The model under review builds one solid part; all positions refer to its coordinate system, in mm. A direction names the side the tool comes from. Coordinates: 2 decimals unless noted, no trailing zeros. Order: outer loops, then holes, each group sorted by start corner. A loop starts at its lowest first (then second) coordinate and runs counter-clockwise, first axis right, second up. Notation, with made-up numbers: (25.5, 27.5) -> (36.5, 27.5) arc R33 ccw to (36.5, 58.5) -> close; hole circle Ø1 at (24.5, 5.5). An arc over 180 degrees is marked (long way). Put each result on its own line as item: value.
from build123d import *

# Parameters (mm, degrees)
SKETCH1_R           = 1.905
BOSS_EXTRUDE1_DEPTH = 0.8001
CIRPATTERN1_COUNT   = 3
SKETCH2_R           = 2.54
CUT_EXTRUDE1_DEPTH  = 2.6002
FILLET1_R           = 6.35


with BuildPart() as part:
    # Sketch1 → Boss-Extrude1 (new body, symmetric)
    with BuildSketch(Plane(origin=(0, 0, 0), x_dir=(1, 0, 0), z_dir=(0, 1, 0))):
        with BuildLine():
            Line((-5.08, 17.78), (-5.08, 0))
            Line((-5.08, 0), (5.08, 0))
            Line((5.08, 0), (5.08, 17.78))
            ThreePointArc((5.08, 17.78), (0, 22.86), (-5.08, 17.78))
        make_face()
        with Locations((0, 17.78)):
            Circle(SKETCH1_R, mode=Mode.SUBTRACT)
    boss_extrude1 = extrude(amount=BOSS_EXTRUDE1_DEPTH, both=True)

    # CirPattern1: Boss-Extrude1 ×3 about axis
    cirpattern1_axis = Axis((0, 0, 0), (0, 1, 0))
    for i in range(1, CIRPATTERN1_COUNT):
        add(boss_extrude1.rotate(cirpattern1_axis, i * 360 / CIRPATTERN1_COUNT))

    # Sketch2 → Cut-Extrude1 (cut, through all)
    with BuildSketch(Plane(origin=(0, 0.8001, 0), x_dir=(1, 0, 0), z_dir=(0, 1, 0))):
        Circle(SKETCH2_R)
    extrude(amount=-CUT_EXTRUDE1_DEPTH, mode=Mode.SUBTRACT)

    # Fillet1
    fillet1_edges = [part.edges().sort_by_distance(p)[0] for p in [
        (5.08, 0, -2.932939367),
        (-5.08, 0, -2.932939367),
        (0, 0, 5.865878735),
    ]]
    fillet(fillet1_edges, radius=FILLET1_R)


solid = part.part
Item 1: For line 1 (X direction, y = -0.3, z = 8); line 2 (X direction, y = 0.3, z = 9); line 3 (Z direction, x = -0.5, y = -0.35), list the stretches that pass through material, from the lowest coordinate up. Write a range as from..to.
Answers below:
line 1: -20.4..-17.08, -13.71..-3.7, 3.7..13.71, 17.08..20.4
line 2: -20.48..-17.3, -13.5..-5.43, 5.43..13.5, 17.3..20.48
line 3: -22.84..-19.62, -15.94..-2.49, 2.49..6.87
Item 2: For pin 1 Ø0.8 at (y, z) = (0, -12.5) entering from -X, flat-tipped, find the tip position at first contact; note if it passes through.
Answers below:
pin 1: x = -5.08
Item 3: For faces 5 (the flat face through (-5.08, 0, -12)), 6 (the flat face through (-3, 0.8, -2)), 7 (the flat face through (5.08, 0, -12)), 8 (the cylindrical face through (16.422, -0.011, 7.284)), 9 (the flat face through (-8.08, 0.01, 10.53)), list the 3-axis set-ups (+Z, -Z, +X, -X, +Y, -Y) from which the entire face can be reached by the end or side of a thin tool; tool diameter is ignored.
Answers below:
face 5: -Z, -X, +Y, -Y
face 6: +Z, -Z, +X, -X, +Y
face 7: -Z, +X, +Y, -Y
face 8: +Y, -Y
face 9: +Z, +Y, -Y
Item 4: Consider section B-B on z = 0. Write out the cut boundary in (x, y), and give its area (3 significant figures).
Answers below:
outline: (-10.16, -0.8) -> (-2.54, -0.8) -> (-2.54, 0.8) -> (-10.16, 0.8) -> close; (2.54, -0.8) -> (10.16, -0.8) -> (10.16, 0.8) -> (2.54, 0.8) -> close
area: 24.4 mm^2
Item 5: Consider section C-C on y = 0.2. Write out the cut boundary in (x, z) (3 decimals).
Answers below:
outline: (-17.938, 4.491) -> (-8.255, -1.1) arc R6.35 cw to (-5.08, -6.599) -> (-5.08, -17.78) arc R5.08 ccw to (5.08, -17.78) -> (5.08, -6.599) arc R6.35 cw to (8.255, -1.1) -> (17.938, 4.491) arc R5.08 ccw to (12.858, 13.289) -> (3.175, 7.699) arc R6.35 cw to (-3.175, 7.699) -> (-12.858, 13.289) arc R5.08 ccw to start; hole circle Ø3.81 at (-15.398, 8.89); hole circle Ø5.08 at (0, 0); hole circle Ø3.81 at (0, -17.78); hole circle Ø3.81 at (15.398, 8.89)
Item 6: Consider section A-A on x = 0. Write out the cut boundary in (y, z) (3 decimals), and give its area (3 significant figures).
Answers below:
outline: (-0.8, -22.86) -> (0.8, -22.86) -> (0.8, -19.685) -> (-0.8, -19.685) -> close; (-0.8, -15.875) -> (0.8, -15.875) -> (0.8, -2.54) -> (-0.8, -2.54) -> close; (-0.8, 2.54) -> (0.8, 2.54) -> (0.8, 6.848) -> (-0.8, 6.848) -> close
area: 33.3 mm^2
Item 7: Consider section D-D on x = -15. Write out the cut boundary in (y, z).
Answers below:
outline: (-0.8, 2.79) -> (0.8, 2.79) -> (0.8, 7.03) -> (-0.8, 7.03) -> close; (-0.8, 10.75) -> (0.8, 10.75) -> (0.8, 13.95) -> (-0.8, 13.95) -> close
Item 8: Mouldability with a two-part tool opening along X and no side actions: class faces 1 (the cylindrical face through (5.954, 0.011, -3.384)), 2 (the flat face through (-13.029, 0.011, 1.656)), 3 (the flat face through (7.949, 0.011, 10.455)), 4 (the cylindrical face through (-0.33, 0.01, -2.52)) as +X half, -X half, draft (parallel to the pull), parting line (faces both ways), or undercut.
Answers below:
face 1: +X half
face 2: -X half
face 3: undercut
face 4: undercut
